Read the model definition and answer for the solid it produces. Units are mm, in the model's axes. A direction names the side the tool comes from. Give positions to 0.01 mm unless a question says otherwise; leave off trailing zeros. Loops run counter-clockwise (first coordinate to the right, second up) from the corner with the lowest first, then second, coordinate; pieces in that order, holes last. Notation, with made-up numbers: (-5.5, -15.5) - (9.5, -15.5) arc R28 ccw to (9.5, 17.5) - close; hole circle Ø9 at (61, -17). An arc over 180 degrees is marked (long way). Put each result on its own line as item: value. Start each with the question number.
1. For faces 1 (the flat face through (58.42, -24, 21)), 2 (the flat face through (29, -1.27, 21)), determine the directions among +Z, -Z, +X, -X, +Y, -Y from which every point of the face is accessible in a straight line to the end or side of a thin tool.
2. A cutting plane is placed at C-C, the plane y = -28.5. Determine the outline of the cut face in (x, z), plus the area to 3 significant figures.
3. A cutting plane is placed at A-A, the plane z = 34.5. Determine the outline of the cut face in (x, y).
4. Consider L1, parallel to X at y = -33.5, z = 37; L2, parallel to Y at x = 26, z = 29; L3, parallel to Z at x = 14.5, y = -25.5. Determine where each line is inside the solid, lowest interval first. Write a range as from..to.
5. Given pin 1 Ø23 at (x, y) = (39, -22) entering from +Z, flat-ended and moving along its own axis, determine where the tip first touches the part or whether it passes through.
6. A cutting plane is placed at B-B, the plane x = 19.5. Determine the outline of the cut face in (y, z).
7. For a pull along X with two mould halves and no side action, classify faces 3 (the flat face through (0, -24, 21)), 4 (the flat face through (57.15, -24, 21)), 5 (the flat face through (26.9, -47.3, 41.91)), 6 (the flat face through (29, -24, 1.27)) as released by +X, released by -X, zero draft, split by the parting line, or undercut.
Autodesk Inventor part; units mm, degrees
ref_plane "YZ Plane" through (0, 0, 0) normal (1, 0, 0) x (0, 1, 0)
ref_plane "XZ Plane" through (0, 0, 0) normal (0, 1, 0) x (-1, 0, 0)
ref_plane "XY Plane" through (0, 0, 0) normal (0, 0, 1) x (1, 0, 0)
sketch "Sketch1" plane through (0, 0, 0) normal (0, 0, 1) x (1, 0, 0)
  line L0 (0, 0) -> (58.42, 0)
  line L1 (58.42, 0) -> (58.42, -48.26)
  line L2 (58.42, -48.26) -> (0, -48.26)
  line L3 (0, -48.26) -> (0, 0)
  dimension "d0" = 58.42
  dimension "d1" = 48.26
extrude "Extrusion1" add sketch "Sketch1" along normal blind 1.27
sketch "Sketch2" plane through (0, 0, 1.27) normal (0, 0, 1) x (1, 0, 0)
  line L0 (58.42, 0) -> (0, 0)
  line L1 (0, 0) -> (0, -48.26)
  line L2 (0, -48.26) -> (58.42, -48.26)
  line L3 (58.42, -48.26) -> (58.42, 0)
  line L4 (1.27, -1.27) -> (57.15, -1.27)
  line L5 (57.15, -1.27) -> (57.15, -46.99)
  line L6 (57.15, -46.99) -> (1.27, -46.99)
  line L7 (1.27, -46.99) -> (1.27, -1.27)
  dimension "d4" = 1.27
  dimension "d5" = 1.27
  dimension "d6" = 1.27
  dimension "d7" = 1.27
extrude "Extrusion2" add sketch "Sketch2" along normal blind 40.64
properties part number "Box Bottom"
Return value:
1. face 1: +Z, -Z, +X, +Y, -Y
1. face 2: +Z
2. outline: (0, 0) - (58.42, 0) - (58.42, 41.91) - (57.15, 41.91) - (57.15, 1.27) - (1.27, 1.27) - (1.27, 41.91) - (0, 41.91) - close
2. area: 177 mm2
3. outline: (0, -48.26) - (58.42, -48.26) - (58.42, 0) - (0, 0) - close; hole (1.27, -46.99) - (57.15, -46.99) - (57.15, -1.27) - (1.27, -1.27) - close
4. L1: x = 0..1.27, 57.15..58.42
4. L2: y = -48.26..-46.99, -1.27..0
4. L3: z = 0..1.27
5. pin 1: stops at z = 1.27
6. outline: (-48.26, 0) - (0, 0) - (0, 41.91) - (-1.27, 41.91) - (-1.27, 1.27) - (-46.99, 1.27) - (-46.99, 41.91) - (-48.26, 41.91) - close
7. face 3: released by -X
7. face 4: undercut
7. face 5: zero draft
7. face 6: undercut
